Autodesk Inventor part; units mm, degrees
ref_plane "Arbeitsebene1" through (0, 3.5, 0) normal (0, 1, 0) x (-1, 0, 0)
ref_plane "YZ Plane" through (0, 0, 0) normal (1, 0, 0) x (0, 1, 0)
ref_plane "XY Plane" through (0, 0, 0) normal (0, 0, 1) x (1, 0, 0)
sketch "Skizze1" plane through (0, 0, 0) normal (0, 1, 0) x (-1, 0, 0)
  line L0 (0, 0) -> (-16.65, 0)
  arc A0 (-16.65, 0) -> (-22.65, 6) centre (-22.65, 0) ccw
  line L1 (-22.65, 6) -> (-34.45, 6)
  arc A1 (-31.15, 9.3) -> (-34.45, 6) centre (-31.15, 6) ccw
  line L2 (-31.15, 9.3) -> (-14.85, 9.3)
  arc A2 (-10.9092, 5.9857) -> (-14.85, 9.3) centre (-14.85, 5.3) ccw
  arc A3 (-10.9092, 5.9857) -> (-7.9536, 3.5) centre (-7.9536, 6.5) ccw
  line L3 (-7.9536, 3.5) -> (0, 3.5)
  line L4 (0, 3.5) -> (0, 0)
  dimension "d0" = 3
  dimension "d1" = 4
  dimension "d2" = 3.5
  dimension "d3" = 7.8
  dimension "d4" = 3.3
  dimension "d5" = 6
  dimension "d6" = 14.85
  dimension "d7" = 19.6
extrude "Extrusion1" add sketch "Skizze1" along normal blind 7
sketch "Skizze3" plane through (0, 0, 0) normal (0, -1, 0) x (1, 0, 0)
  arc A0 (14.85, 9.3) -> (10.9092, 5.9857) centre (14.85, 5.3) ccw
  point P0 (0, 0)
hole "Bohrung1" at (14.85, 0, 5.3) direction (0, 1, 0) diameter 4 depth 7
sketch "Skizze4" plane through (14.85, 0, 9.3) normal (0, 0, 1) x (1, 0, 0)
  line L0 (-2, 7) -> (2, 7)
  line L1 (2, 0) -> (-2, 0)
  line L2 (0, 0) -> (0, 7) construction
  line L3 (0, 7) -> (0, 0) construction
  line L4 (1.8, 0) -> (-14.85, 0)
  arc A0 (-4.75, 0) -> (-7.25, 0) centre (-6, 0) ccw
  dimension "d17" = 1.25
  dimension "d18" = 6
extrude "Extrusion2" cut sketch "Skizze4" against normal up to surface (9.3 mm away)
fillet "Rundung1" radius 1.25 2 edges at (10.1, 0, 2.202) (7.6, 0, 1.75)
ref_plane "Arbeitsebene1" through (0, 3.5, 0) normal (0, 1, 0) x (-1, 0, 0)
mirror "Spiegeln1" about plane through (0, 3.5, 0) normal (0, 1, 0) of "Extrusion2", "Rundung1"
fillet "Rundung2" radius 3.5 2 edges at (0, 0, 1.75) (0, 7, 1.75)
sketch "Skizze5" plane through (7.9536, 0.8712, 3.5) normal (0, 0, 1) x (1, 0, 0)
  arc A0 (-4.4536, 6.1288) -> (-4.4536, -0.8712) centre (-4.4536, 2.6288) ccw
  point P0 (-7.9536, -0.8712)
hole "Bohrung2" at (3.5, 3.5, 3.5) direction (0, 0, -1) diameter 4.5 depth 3.5
sketch "Skizze6" plane through (14.85, 0, 9.3) normal (0, 0, 1) x (1, 0, 0)
  line L0 (0, 0) -> (16.3, 0)
  line L1 (16.3, 0) -> (16.3, 7)
  line L2 (0, 7) -> (16.3, 7)
  line L3 (0, 0) -> (0, 7)
  line L4 (16.3, 0) -> (19.6, 0)
  line L5 (19.6, 0) -> (19.6, 7)
  line L6 (16.3, 7) -> (19.6, 7)
  line L7 (16.3, 0) -> (16.3, 7)
  line L8 (8, 5.5) -> (19.6, 5.5)
  line L9 (8, 5.5) -> (8, 7)
  point P0 (-14.85, 0)
  point P1 (8, 6.25)
  dimension "d32" = 1.5
  dimension "d38" = 8
extrude "Extrusion5" cut sketch "Skizze6" against normal up to surface (3.3 mm away) contours L8 L9 L2 L1 | L1 L6 L5 L8
mirror "Spiegeln2" about plane through (0, 3.5, 0) normal (0, 1, 0) of "Extrusion5"
fillet "Rundung3" radius 2 2 edges at (22.85, 5.5, 7.65) (22.85, 1.5, 7.65)
properties part number "KippHebel" material "Blei"
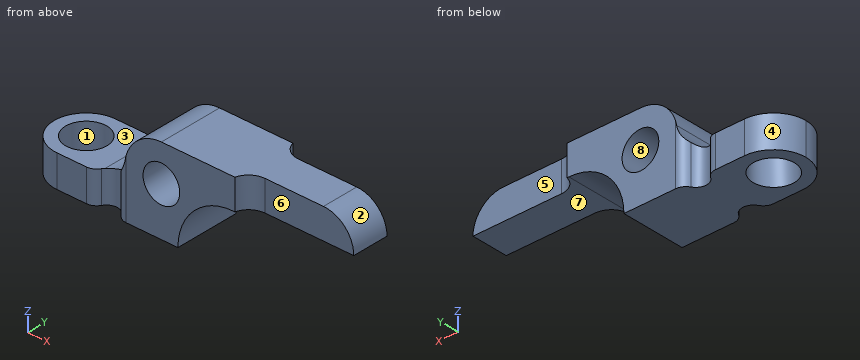
Can you work these out from the model? Positions are in its coordinate system, mm. Face numbers are marked on the shaded views. A direction names the side the tool comes from. Give positions to 0.01 mm unless a question says otherwise; leave off trailing zeros. Order: outer loops, then holes, each group sorted by start corner. A loop starts at its lowest first (then second) coordinate and runs counter-clockwise, first axis right, second up. Notation, with made-up numbers: (-0.5, 8.5) - (44.5, 8.5) arc R5 cw to (44.5, 17.5) - close; hole circle Ø5 at (63, 7). An arc over 180 degrees is marked (long way). Use a Markdown table: item, result. Add a question column.
Q1. If we mould it in two halves opening along X, with no side actions, what happens to the marked faces 1, 2, 3 and 4? For each: released by +X, released by -X, zero draft, split by the parting line, or undercut.
Q2. If we section it at B-B on z = 7: Write out the boundary of the cut face in (x, y).
Q3. If we section it at C-C on x = 2: Write out the boundary of the cut face in (y, z), plus the area to 3 significant figures.
Q4. If we section it at A-A on y = 5: Write out the boundary of the cut face in (x, z).
Q5. If we section it at D-D on z = 5.3: Write out the boundary of the cut face in (x, y).
Q6. Please list where these lines run through material, in increasing order: line 1 along Y through (x, z) = (3.5, 1.95); line 2 along Z through (x, y) = (14.85, 2); line 3 along X through (y, z) = (3.5, 6.5).
Q7. I'm going to push flat-ended pins straight in: pin 1 (3.5 mm diameter, centred on x = 31, y = 4, fed in from -Z); pin 2 (1 mm diameter, centred on y = 1.5, z = 1, fed in from +X); pin 3 (3.5 mm diameter, centred on x = 14.85, z = 5.3, fed in from +Y); pin 4 (1 mm diameter, centred on y = 5.5, z = 3.5, fed in from +X). Where does each tip first touch, or does it pass through?
Q8. On a 3-axis mill with a long thin cutter (end or side, diameter ignored), from which of +Z, -Z, +X, -X, +Y, -Y can I reach the whole of each face in a straight line? I mean the marked faces 5, 6, 7 and 8. Say none if no direction works.
Answers follow:
| question | item | result |
|---|---|---|
| 1 | face 1 | undercut |
| 1 | face 2 | released by +X |
| 1 | face 3 | zero draft |
| 1 | face 4 | released by -X |
| 2 | outline | (11.23, 0) - (13.8, 0) - (13.8, 7) - (11.23, 7) - close; (15.9, 0) - (22.85, 0) arc R2 cw to (24.79, 1.5) - (34.29, 1.5) - (34.29, 5.5) - (24.79, 5.5) arc R2 cw to (22.85, 7) - (15.9, 7) - close |
| 3 | outline | (0.34, 0) - (1.82, 0) - (1.82, 3.5) - (0.34, 3.5) - close; (5.18, 0) - (6.66, 0) - (6.66, 3.5) - (5.18, 3.5) - close |
| 3 | area | 10.4 mm^2 |
| 4 | outline | (0.34, 0) - (1.82, 0) - (1.82, 3.5) - (0.34, 3.5) - close; (5.18, 0) - (16.65, 0) arc R6 cw to (22.65, 6) - (34.45, 6) arc R3.3 ccw to (31.15, 9.3) - (14.85, 9.3) arc R4 ccw to (10.91, 5.99) arc R3 cw to (7.95, 3.5) - (5.18, 3.5) - close; hole circle Ø4 at (14.85, 5.3) |
| 5 | outline | (10.7, 0.04) arc R1.25 ccw to (11.02, 0) - (12.85, 0) - (12.85, 7) - (11.02, 7) arc R1.25 ccw to (10.7, 6.96) - close; (16.85, 0) - (19.84, 0) - (19.84, 7) - (16.85, 7) - close |
| 6 | line 1 | y = 0 to 1.25, 5.75 to 7 |
| 6 | line 2 | z = 0 to 3.3, 7.3 to 9.3 |
| 6 | line 3 | x = 11.03 to 13.25, 16.45 to 34.41 |
| 7 | pin 1 | stops at z = 6 |
| 7 | pin 2 | stops at x = 16.84 |
| 7 | pin 3 | passes through |
| 7 | pin 4 | stops at x = 18.18 |
| 8 | face 5 | +Z, -Z, +X, +Y |
| 8 | face 6 | +Z, -Z, +X, -Y |
| 8 | face 7 | -Z, +X, +Y, -Y |
| 8 | face 8 | +Y, -Y |
